Autodesk Fusion 360 part; units mm, degrees
sketch "スケッチ1" plane through (0, 0, 0) normal (0, 0, 1) x (1, 0, 0)
  line L0 (0, 0) -> (36, 0)
  line L1 (36, 0) -> (36, 34)
  line L2 (36, 34) -> (0, 34)
  line L3 (0, 34) -> (0, 0)
  line L4 (0, 34) -> (0, 17)
  line L5 (0, 17) -> (5, 17)
  circle A0 centre (5, 17) radius 1.5
  line L6 (5, 17) -> (31, 17)
  circle A1 centre (31, 17) radius 1.5
  line L7 (31, 17) -> (36, 17)
  dimension "d1" = 36
  dimension "d2" = 34
  dimension "d3" = 3
  dimension "d4" = 26
  dimension "d5" = 3
extrude "押し出し1" add sketch "スケッチ1" along normal blind 1 contours L0 L1 L3 L5 A0 L6 A1 L7 | L1 L2 L3 L4 L5 A0 L6 A1 L7
Source: CAD feature listing. Evaluate the final solid. Frame: model axes, mm. Give positions to 0.01 mm unless a question says otherwise; leave off trailing zeros. Loops run counter-clockwise (first coordinate to the right, second up) from the corner with the lowest first, then second, coordinate; pieces in that order, holes last. Notation, with made-up numbers: (49.25, 88.25) -> (90.25, 88.25) arc R23 cw to (90.25, 100.25) -> close; hole circle Ø4 at (70.25, 64.25). An arc over 180 degrees is marked (long way). Use a Markdown table: item, result. Add a question column.
(1) Section query B-B (x = 5). Output: boundary loops of the cut face in (y, z), then the cut area to 3 significant figures.
(2) Section query A-A (y = 17). Output: boundary loops of the cut face in (x, z), then the cut area to 3 significant figures.
(3) Pull-direction query (Y, two-part tool) for faces 1 (the face through (17.7, 0, 0.5)), 2 (the face through (36, 16.8, 0.5)), 3 (the face through (5.806, 15.735, 0.493)); classes: +Y half, -Y half, draft (parallel to the pull), parting line (faces both ways), or undercut.
(4) Ray query, line 1 (X direction, y = 17, z = 0.3); line 2 (Y direction, x = 31, z = 0.7); line 3 (X direction, y = 16, z = 0.75). Return the intervals inside material, ascending.
Checked values:
| question | item | result |
|---|---|---|
| 1 | outline | (0, 0) -> (15.5, 0) -> (15.5, 1) -> (0, 1) -> close; (18.5, 0) -> (34, 0) -> (34, 1) -> (18.5, 1) -> close |
| 1 | area | 31.0 mm^2 |
| 2 | outline | (0, 0) -> (3.5, 0) -> (3.5, 1) -> (0, 1) -> close; (6.5, 0) -> (29.5, 0) -> (29.5, 1) -> (6.5, 1) -> close; (32.5, 0) -> (36, 0) -> (36, 1) -> (32.5, 1) -> close |
| 2 | area | 30.0 mm^2 |
| 3 | face 1 | -Y half |
| 3 | face 2 | draft |
| 3 | face 3 | undercut |
| 4 | line 1 | 0 to 3.5, 6.5 to 29.5, 32.5 to 36 |
| 4 | line 2 | 0 to 15.5, 18.5 to 34 |
| 4 | line 3 | 0 to 3.88, 6.12 to 29.88, 32.12 to 36 |
